from build123d import *

# Parameters (mm, degrees)
SKETCH1_W                = 42.3
SKETCH1_H                = 42.3
BOSS_EXTRUDE1_DEPTH      = 40
SKETCH1_3_R              = 1.5
CUT_EXTRUDE1_DEPTH       = 5
SKETCH1_4_R              = 11.25
SKETCH1_4_R_2            = 2.5
BOSS_EXTRUDE2_DEPTH      = 1.5
BOSS_EXTRUDE3_DEPTH      = 25
BOSS_EXTRUDE3_DEPTH_BACK = 40
BOSS_EXTRUDE3_START      = 1.5
SKETCH1_5_R              = 2.5
SKETCH3_W                = 17
SKETCH3_H                = 9
BOSS_EXTRUDE4_DEPTH      = 5


with BuildPart() as part:
    # Sketch1 → Boss-Extrude1 (new body)
    with BuildSketch(Plane.XY):
        Rectangle(SKETCH1_W, SKETCH1_H)
    extrude(amount=-BOSS_EXTRUDE1_DEPTH)

    # Sketch1<3> → Cut-Extrude1 (cut)
    with BuildSketch(Plane.XY):
        with Locations((-15.5, -15.5)):
            Circle(SKETCH1_3_R)
        with Locations((15.5, 15.5)):
            Circle(SKETCH1_3_R)
        with Locations((15.5, -15.5)):
            Circle(SKETCH1_3_R)
        with Locations((-15.5, 15.5)):
            Circle(SKETCH1_3_R)
    extrude(amount=-CUT_EXTRUDE1_DEPTH, mode=Mode.SUBTRACT)

    # Sketch1<4> → Boss-Extrude2 (add)
    with BuildSketch(Plane.XY):
        Circle(SKETCH1_4_R)
        Circle(SKETCH1_4_R_2, mode=Mode.SUBTRACT)
    extrude(amount=BOSS_EXTRUDE2_DEPTH)

    # Sketch1<5> → Boss-Extrude3 (add, two sides: drawn at the far end of the back side and taken through both)
    with BuildSketch(Plane.XY.offset(BOSS_EXTRUDE3_START - BOSS_EXTRUDE3_DEPTH_BACK)):
        Circle(SKETCH1_5_R)
    extrude(amount=BOSS_EXTRUDE3_DEPTH + BOSS_EXTRUDE3_DEPTH_BACK)

    # Sketch3 → Boss-Extrude4 (add)
    with BuildSketch(Plane.XZ.offset(21.15)):
        with Locations((0, -35.5)):
            Rectangle(SKETCH3_W, SKETCH3_H)
    extrude(amount=BOSS_EXTRUDE4_DEPTH)


solid = part.part
Part model, mm, in its own coordinate system. A direction names the side the tool comes from. Coordinates: 2 decimals unless noted, no trailing zeros. Loops run counter-clockwise (first coordinate to the right, second up) from the corner with the lowest first, then second, coordinate; pieces in that order, holes last. Notation, with made-up numbers: (-35, 64.5) - (-12, 64.5) arc R27 cw to (-12, 101.5) - close; hole circle Ø11 at (82, 58). An arc over 180 degrees is marked (long way). Write each question's results on one line, items separated by ' | '. Start each with the question number.
Q1. Slice it at A-A on x = 0. Give the cut face in (y, z).
Q2. Probe line 1 along Y through (x, z) = (15.5, -2.2); line 2 along X through (y, z) = (-15, -3). List the from-to ranges inside material, lowest first.
Q3. Slice it at B-B on y = 15.5. Give the cut face in (x, z).
Q4. Which spindle directions (+Z, -Z, +X, -X, +Y, -Y) get a long thin tool onto all of the face, cutting with end or side? Do faces 4 (the flat face through (0, -24, -31)), 5 (the flat face through (0, -2, -40)), 6 (the flat face through (8.5, -24, -36)), 7 (the cylindrical face through (-17, 15.57, -2.46)). Say none if no direction does.
Q5. Drop flat-ended pins along their axis: pin 1 Ø4 at (y, z) = (-5, 16) entering from +X; pin 2 Ø3.5 at (x, y) = (-15.5, 15) entering from +Z; pin 3 Ø1.8 at (x, y) = (15.5, -15.5) entering from +Z; pin 4 Ø2.5 at (x, y) = (-4, -24.5) entering from +Z. Give the stop position or say it passes through.
Q6. Slice it at C-C on z = -22. Give the cut face in (x, y), and give its area (3 significant figures).
Q7. Two-plate mould, pull along X, no slides. Class faces 1 (the flat face through (21.15, 0, -20)), 2 (the flat face through (0, 21.15, -20)), 3 (the flat face through (15, -15, -5)): +X half, -X half, draft (parallel to the pull), parting line (faces both ways), or undercut.
Answer:
1) outline: (-26.15, -40) - (21.15, -40) - (21.15, 0) - (11.25, 0) - (11.25, 1.5) - (2.5, 1.5) - (2.5, 26.5) - (-2.5, 26.5) - (-2.5, 1.5) - (-11.25, 1.5) - (-11.25, 0) - (-21.15, 0) - (-21.15, -31) - (-26.15, -31) - close
2) line 1: y = -21.15 to -17, -14 to 14, 17 to 21.15 | line 2: x = -21.15 to -16.91, -14.09 to 14.09, 16.91 to 21.15
3) outline: (-21.15, -40) - (21.15, -40) - (21.15, 0) - (17, 0) - (17, -5) - (14, -5) - (14, 0) - (-14, 0) - (-14, -5) - (-17, -5) - (-17, 0) - (-21.15, 0) - close
4) face 4: +Z, +X, -X, -Y | face 5: -Z, +X, -X, +Y, -Y | face 6: +Z, -Z, +X, -Y | face 7: +Z
5) pin 1: passes through | pin 2: stops at z = 0 | pin 3: stops at z = -5 | pin 4: stops at z = -31
6) outline: (-21.15, -21.15) - (21.15, -21.15) - (21.15, 21.15) - (-21.15, 21.15) - close | area: 1,790 mm2
7) face 1: +X half | face 2: draft | face 3: undercut
